Design review of the part built by this model. Coordinates are the model's own, in mm. A direction names the side the tool comes from. Give positions to 0.01 mm unless a question says otherwise; leave off trailing zeros. Write each loop counter-clockwise with the first axis right and the second up, starting at its lowest first coordinate (ties: lowest second). Pieces come first, ordered by that corner, then holes. Notation, with made-up numbers: M 5.5,85 L 25.5,85 A15 ccw 25.5,108 Z; hole C 8,-6.5 d4. An arc over 180 degrees is marked long. Write each question's results on one line, items separated by ' | '. Start each with the question number.
from build123d import *

# Parameters (mm, degrees)
ESQUISSE1_W                  = 150
ESQUISSE1_H                  = 150
BOSS_EXTRU_1_DEPTH           = 25
CHANFREIN1_SIZE              = 25
CHANFREIN1_SIZE_2            = 6.5
ESQUISSE2_W                  = 137
ESQUISSE2_H                  = 137
ESQUISSE2_W_2                = 10
ESQUISSE2_H_2                = 10
ESQUISSE2_W_3                = 60
ESQUISSE2_H_3                = 58
ESQUISSE2_R                  = 1.75
ENL_V_MAT_EXTRU_2_DEPTH      = 15
ESQUISSE3_W                  = 12.5
ESQUISSE3_H                  = 18
ENL_V_MAT_EXTRU_3_DEPTH      = 15
ENL_V_MAT_EXTRU_4_DEPTH      = 20
ENL_V_MAT_EXTRU_4_DEPTH_BACK = 2
ESQUISSE5_W                  = 60
ESQUISSE5_H                  = 58
ESQUISSE5_W_2                = 56
ESQUISSE5_H_2                = 54
ENL_V_MAT_EXTRU_7_DEPTH      = 8
ESQUISSE6_W                  = 56
ESQUISSE6_H                  = 54
ENL_V_MAT_EXTRU_6_DEPTH      = 22
ESQUISSE7_W                  = 8
ESQUISSE7_H                  = 4
ENL_V_MAT_EXTRU_13_DEPTH     = 8
ESQUISSE8_R                  = 2.14482531
ENL_V_MAT_EXTRU_9_DEPTH      = 8
ESQUISSE9_R                  = 4.485216979
ESQUISSE9_R_2                = 4.690098516
ESQUISSE9_R_3                = 4.770954249
ESQUISSE9_R_4                = 4.498432912
ENL_V_MAT_EXTRU_10_DEPTH     = 22
ESQUISSE10_W                 = 6.913683137
ESQUISSE10_H                 = 8.110809872
ENL_V_MAT_EXTRU_11_DEPTH     = 8
ESQUISSE11_W                 = 10
ESQUISSE11_H                 = 4
ENL_V_MAT_EXTRU_12_DEPTH     = 8


with BuildPart() as part:
    # Esquisse1 → Boss.-Extru.1 (new body)
    with BuildSketch(Plane.XY):
        with Locations((75, 75)):
            Rectangle(ESQUISSE1_W, ESQUISSE1_H)
    extrude(amount=BOSS_EXTRU_1_DEPTH)

    # Chanfrein1
    # the kernel refuses this chamfer: 25, 6.5 mm, written as the material it takes off along each edge
    with BuildSketch(Plane(origin=(150, -64.922604179, 25), x_dir=(0.00968976271621493, 0, -0.9999530531472482), z_dir=(0, 1, 0)), Plane(origin=(214.922604179, 150, 25), x_dir=(0, 0.00968976271621493, -0.9999530531472482), z_dir=(-1, 0, 0)), Plane(origin=(0, 214.922604179, 25), x_dir=(-0.009689762716214955, 0, -0.9999530531472482), z_dir=(0, -1, 0)), Plane(origin=(-64.922604179, 0, 25), x_dir=(0, -0.009689762716214955, -0.9999530531472482), z_dir=(1, 0, 0))) as chanfrein1_piece_1:
        Polygon((CHANFREIN1_SIZE * 0.999953053147, CHANFREIN1_SIZE * 0.00968976271621), (-CHANFREIN1_SIZE_2 * 0.00968976271621, CHANFREIN1_SIZE_2 * 0.999953053147), (0, 0), align=None)
    extrude(amount=279.845208358, mode=Mode.SUBTRACT)

    # Esquisse2 → Enlèv. mat.-Extru.2 (cut)
    # profile 1 of 5: a face of its own
    with BuildSketch(Plane.XY.offset(25)):
        with Locations((75, 75)):
            Rectangle(ESQUISSE2_W, ESQUISSE2_H)
        with Locations((14.7, 14.7)):
            Rectangle(ESQUISSE2_W_2, ESQUISSE2_H_2, mode=Mode.SUBTRACT)
        with Locations((135.3, 14.7)):
            Rectangle(ESQUISSE2_W_2, ESQUISSE2_H_2, mode=Mode.SUBTRACT)
        with Locations((93.5, 74.5)):
            Rectangle(ESQUISSE2_W_3, ESQUISSE2_H_3, mode=Mode.SUBTRACT)
        with Locations((14.7, 135.3)):
            Rectangle(ESQUISSE2_W_2, ESQUISSE2_H_2, mode=Mode.SUBTRACT)
        with Locations((135.3, 135.3)):
            Rectangle(ESQUISSE2_W_2, ESQUISSE2_H_2, mode=Mode.SUBTRACT)
    # profile 2 of 5: a face of its own
    with BuildSketch(Plane.XY.offset(25)):
        with Locations((14.7, 135.3)):
            Circle(ESQUISSE2_R)
    # profile 3 of 5: a face of its own
    with BuildSketch(Plane.XY.offset(25)):
        with Locations((135.3, 135.3)):
            Circle(ESQUISSE2_R)
    # profile 4 of 5: a face of its own
    with BuildSketch(Plane.XY.offset(25)):
        with Locations((135.3, 14.7)):
            Circle(ESQUISSE2_R)
    # profile 5 of 5: a face of its own
    with BuildSketch(Plane.XY.offset(25)):
        with Locations((14.7, 14.7)):
            Circle(ESQUISSE2_R)
    extrude(amount=-ENL_V_MAT_EXTRU_2_DEPTH, mode=Mode.SUBTRACT)

    # Esquisse3 → Enlèv. mat.-Extru.3 (cut)
    with BuildSketch(Plane(origin=(140.502060697, 0, 36.530535781), x_dir=(0.2516338517649486, 0, -0.9678225067882726), z_dir=(0.9678225067882725, 0, 0.25163385176494857))):
        with Locations((24.495077765, 117.5)):
            Rectangle(ESQUISSE3_W, ESQUISSE3_H)
    extrude(amount=-ENL_V_MAT_EXTRU_3_DEPTH, mode=Mode.SUBTRACT)

    # Esquisse4 → Enlèv. mat.-Extru.4 (cut, two sides: drawn at the far end of the back side and taken through both)
    with BuildSketch(Plane(origin=(0, 108.5, 0), x_dir=(1, 0, 0), z_dir=(0, 1, 0)).offset(-ENL_V_MAT_EXTRU_4_DEPTH_BACK)):
        Polygon((146.541727915, -8.467609261), (144.547390296, -16.138138565), (141.512044488, -15.348948655), (143.506382107, -7.678419351), align=None)
    extrude(amount=ENL_V_MAT_EXTRU_4_DEPTH + ENL_V_MAT_EXTRU_4_DEPTH_BACK, mode=Mode.SUBTRACT)

    # Esquisse5 → Enlèv. mat.-Extru.7 (cut)
    # profile 1 of 2: a face of its own
    with BuildSketch(Plane(origin=(0, 0, 0), x_dir=(-1, 0, 0), z_dir=(0, 0, -1))):
        Polygon((-125.912264941, 103.398684795), (-125.912264941, 143.5), (-25.60196638, 143.5), (-25.60196638, 125.072705698), (-6.5, 125.072705698), (-6.5, 27.173820188), (-25.60196638, 27.173820188), (-25.60196638, 6.5), (-125.912264941, 6.5), (-125.912264941, 27.173820188), (-143.5, 27.173820188), (-143.5, 103.398684795), align=None)
        with Locations((-93.5, 74.5)):
            Rectangle(ESQUISSE5_W, ESQUISSE5_H, mode=Mode.SUBTRACT)
    # profile 2 of 2: a face of its own
    with BuildSketch(Plane(origin=(0, 0, 0), x_dir=(-1, 0, 0), z_dir=(0, 0, -1))):
        with Locations((-93.5, 74.5)):
            Rectangle(ESQUISSE5_W_2, ESQUISSE5_H_2)
    extrude(amount=-ENL_V_MAT_EXTRU_7_DEPTH, mode=Mode.SUBTRACT)

    # Esquisse6 → Enlèv. mat.-Extru.6 (cut)
    with BuildSketch(Plane(origin=(0, 0, 0), x_dir=(-1, 0, 0), z_dir=(0, 0, -1))):
        with Locations((-93.5, 74.5)):
            Rectangle(ESQUISSE6_W, ESQUISSE6_H)
    extrude(amount=-ENL_V_MAT_EXTRU_6_DEPTH, mode=Mode.SUBTRACT)

    # Esquisse7 → Enlèv. mat.-Extru.13 (cut)
    with BuildSketch(Plane.XZ.offset(-101.640366459)):
        with Locations((74.5, 4)):
            Rectangle(ESQUISSE7_W, ESQUISSE7_H)
        with Locations((112.5, 4)):
            Rectangle(ESQUISSE7_W, ESQUISSE7_H)
    extrude(amount=-ENL_V_MAT_EXTRU_13_DEPTH, mode=Mode.SUBTRACT)

    # Esquisse8 → Enlèv. mat.-Extru.9 (cut)
    with BuildSketch(Plane(origin=(0, 103.5, 0), x_dir=(1, 0, 0), z_dir=(0, 1, 0))):
        with Locations(Location((111.298002562, -13.017125877, 0), (0, 0, 180))):
            Circle(ESQUISSE8_R)
    extrude(amount=-ENL_V_MAT_EXTRU_9_DEPTH, mode=Mode.SUBTRACT)

    # Esquisse9 → Enlèv. mat.-Extru.10 (cut)
    with BuildSketch(Plane(origin=(0, 0, 0), x_dir=(-1, 0, 0), z_dir=(0, 0, -1))):
        with Locations((-135.3, 135.3)):
            Circle(ESQUISSE9_R)
        with Locations((-14.7, 135.3)):
            Circle(ESQUISSE9_R_2)
        with Locations((-14.7, 14.7)):
            Circle(ESQUISSE9_R_3)
        with Locations((-135.3, 14.7)):
            Circle(ESQUISSE9_R_4)
    extrude(amount=-ENL_V_MAT_EXTRU_10_DEPTH, mode=Mode.SUBTRACT)

    # Esquisse10 → Enlèv. mat.-Extru.11 (cut)
    with BuildSketch(Plane.XY.offset(10)):
        with Locations((130.264383867, 114.747246467)):
            Rectangle(ESQUISSE10_W, ESQUISSE10_H)
    extrude(amount=-ENL_V_MAT_EXTRU_11_DEPTH, mode=Mode.SUBTRACT)

    # Esquisse11 → Enlèv. mat.-Extru.12 (cut)
    with BuildSketch(Plane(origin=(0, 47.359633541, 0), x_dir=(1, 0, 0), z_dir=(0, 1, 0))):
        with Locations((94.5, -4)):
            Rectangle(ESQUISSE11_W, ESQUISSE11_H)
    extrude(amount=-ENL_V_MAT_EXTRU_12_DEPTH, mode=Mode.SUBTRACT)


solid = part.part
Q1. For pin 1 Ø3 at (x, y) = (34, 100.5) entering from -Z; pin 2 Ø3 at (y, z) = (16.5, 19) entering from +X; pin 3 Ø1.5 at (y, z) = (102, 4.5) entering from -X (3 decimals), all flat-tipped, find the tip position at first contact; note any pin that passes through.
Q2. We need section A-A on y = 14.7. Count the separate pieces of the cut face and the enclosed holes in it, and give its area (3 significant figures).
Q3. For faces 1 (the flat face through (135.2, 12.5, 25)), 2 (the flat face through (144, 128.5, 12)), 3 (the cylindrical face through (12.536, 131.139, 10.846)), 4 (the cylindrical face through (15.51, 133.75, 23.52)), 5 (the flat face through (130.3, 135, 18)), list the 3-axis set-ups (+Z, -Z, +X, -X, +Y, -Y) from which the entire face can be reached by the end or side of a thin tool; tool diameter is ignored.
Q4. The part is to be moulded in two halves that separate along Y. For faces 6 (the flat face through (140, 126.5, 8)), 7 (the flat face through (3.2, 76, 12.3)), say which applies: pulls with the +Y half, pulls with the -Y half, needs draft (parallel to the pull), parting line crosses it, or undercut.
Q5. We need section C-C on y = 35. Write out the cut boundary in (x, z).
Q6. Wall thickness on line 1 along X through (y, z) = (135.3, 23.7); line 2 along X through (y, z) = (90.5, 6.75) (3 decimals); line 3 along Y through (x, z) = (14.7, 15.5): over which ranges is each line inside the solid? List them lowest first. Write a range as from..to.
Answer sheet:
1) pin 1: z = 8 | pin 2: x = 145.45 | pin 3: x = 0.975
2) separate pieces: 3 | enclosed holes: 0 | area: 601 mm^2
3) face 1: +Z, +X, -X, +Y, -Y | face 2: none | face 3: -Z | face 4: +Z, -Z | face 5: +Z
4) face 6: undercut | face 7: needs draft
5) outline: M 0,0 L 6.5,0 L 6.5,8 L 143.5,8 L 143.5,0 L 150,0 L 143.5,25 L 143.5,10 L 6.5,10 L 6.5,25 Z
6) line 1: 6.16..6.5, 9.7..12.95, 16.45..19.7, 130.3..133.55, 137.05..140.3, 143.5..143.84 | line 2: 1.755..6.5, 63.5..65.5, 121.5..123.5, 143.5..148.245 | line 3: 4.03..6.5, 9.7..9.93, 19.47..19.7, 130.3..130.61, 139.99..140.3, 143.5..145.97
